Model file for the job. Use its own axes, mm. Face numbers are marked on the shaded views. A direction names the side the tool comes from. Round coordinates to 2 decimals unless told otherwise and drop trailing zeros. Order: outer loops, then holes, each group sorted by start corner. A loop starts at its lowest first (then second) coordinate and runs counter-clockwise, first axis right, second up. Notation, with made-up numbers: (-10.75, 65.25) -> (28.25, 65.25) arc R21 cw to (28.25, 102.25) -> close; hole circle Ø3 at (3, 5). An arc over 180 degrees is marked (long way). Put each result on its own line as item: value. Start each with the question number.
Q1. Cut at C-C, the plane y = -6.25. List the corners of the cut face in (x, z).
Q2. Pull direction Y, two halves, no side cores. Call the marked faces 4, 5 and 6: released by +Y, released by -Y, zero draft, split by the parting line, or undercut.
Q3. Cut at A-A, the plane z = 2.6. State how many separate pieces and enclosed holes the cut face has, and give its area (3 significant figures).
Q4. Flat gauge pins, fed straight in: P1, Ø3.5, axis at x = 4.5, y = 0, coming from the -Z side; P2, Ø3, axis at x = 30.75, y = 0, coming from the +Z side; P3, Ø2, axis at x = 18.5, z = 2, coming from the -Y side; P4, Ø2, axis at y = -10, z = 2.5, coming from the +X side. Where does each tip first touch, or does it go through?
Q5. 3-axis set-ups, long thin cutter, end or side, ignore diameter. For the marked faces 1, 2 and 3: which of +Z, -Z, +X, -X, +Y, -Y reach the whole face in a straight line?
Q6. Cut at B-B, the plane x = 18.5. List the corners of the cut face in (y, z).
Q7. Probe L1, parallel to Y at x = 0, z = 1.85; L2, parallel to X at y = -13, z = 2.95; L3, parallel to Y at x = -11.5, z = 0.6. List the from-to ranges inside material, lowest first.
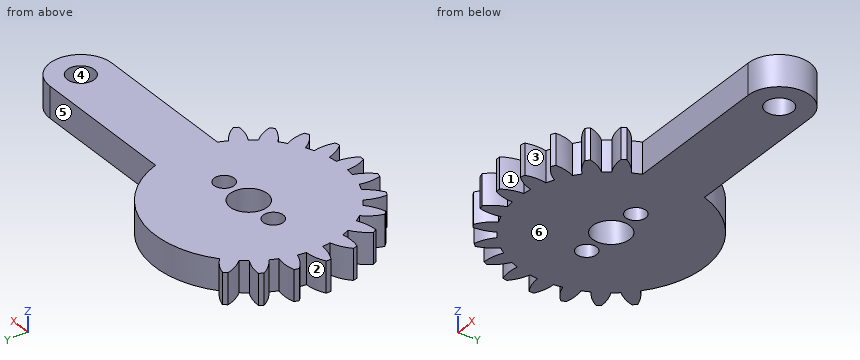
from build123d import *

# Parameters (mm, degrees)
SKETCH1_R           = 1.75
BOSS_EXTRUDE3_DEPTH = 4
SKETCH3_R           = 1.3
SKETCH3_R_2         = 2.4
CUT_EXTRUDE1_DEPTH  = 38.915688046


with BuildPart() as part:
    # Sketch1 → Boss-Extrude3 (new body)
    with BuildSketch(Plane.XY):
        with BuildLine():
            ThreePointArc((11.398526221, 4), (3.187763399, 11.651805204), (-7.774744082, 9.245526186))
            ThreePointArc((-7.774744082, 9.245526186), (-8.865739978, 10.052419077), (-10.123446462, 10.561852666))
            ThreePointArc((-10.123446462, 10.561852666), (-10.344972209, 10.344972209), (-10.561852666, 10.123446462))
            ThreePointArc((-10.561852666, 10.123446462), (-10.052419077, 8.865739978), (-9.245526186, 7.774744082))
            ThreePointArc((-9.245526186, 7.774744082), (-9.583708351, 7.353838062), (-9.90274436, 6.918240682))
            ThreePointArc((-9.90274436, 6.918240682), (-11.16540472, 7.415268848), (-12.51210701, 7.581825517))
            ThreePointArc((-12.51210701, 7.581825517), (-12.669951657, 7.315), (-12.82210701, 7.044889767))
            ThreePointArc((-12.82210701, 7.044889767), (-12.004513558, 5.961889707), (-10.94274436, 5.116907842))
            ThreePointArc((-10.94274436, 5.116907842), (-11.160464753, 4.622815863), (-11.355888976, 4.119488508))
            ThreePointArc((-11.355888976, 4.119488508), (-12.704165582, 4.272780301), (-14.048088143, 4.085109489))
            ThreePointArc((-14.048088143, 4.085109489), (-14.131494839, 3.78652263), (-14.208555951, 3.486235477))
            ThreePointArc((-14.208555951, 3.486235477), (-13.138520279, 2.651746506), (-11.89423259, 2.110362789))
            ThreePointArc((-11.89423259, 2.110362789), (-11.976653925, 1.576756402), (-12.035148524, 1.04))
            ThreePointArc((-12.035148524, 1.04), (-13.377158555, 0.839108838), (-14.626715284, 0.31))
            ThreePointArc((-14.626715284, 0.31), (-14.63, 0), (-14.626715284, -0.31))
            ThreePointArc((-14.626715284, -0.31), (-13.377158555, -0.839108838), (-12.035148524, -1.04))
            ThreePointArc((-12.035148524, -1.04), (-11.976653925, -1.576756402), (-11.89423259, -2.110362789))
            ThreePointArc((-11.89423259, -2.110362789), (-13.138520279, -2.651746506), (-14.208555951, -3.486235477))
            ThreePointArc((-14.208555951, -3.486235477), (-14.131494839, -3.78652263), (-14.048088143, -4.085109489))
            ThreePointArc((-14.048088143, -4.085109489), (-12.704165582, -4.272780301), (-11.355888976, -4.119488508))
            ThreePointArc((-11.355888976, -4.119488508), (-11.160464753, -4.622815863), (-10.94274436, -5.116907842))
            ThreePointArc((-10.94274436, -5.116907842), (-12.004513558, -5.961889707), (-12.82210701, -7.044889767))
            ThreePointArc((-12.82210701, -7.044889767), (-12.669951657, -7.315), (-12.51210701, -7.581825517))
            ThreePointArc((-12.51210701, -7.581825517), (-11.16540472, -7.415268848), (-9.90274436, -6.918240682))
            ThreePointArc((-9.90274436, -6.918240682), (-9.583708351, -7.353838062), (-9.245526186, -7.774744082))
            ThreePointArc((-9.245526186, -7.774744082), (-10.052419077, -8.865739978), (-10.561852666, -10.123446462))
            ThreePointArc((-10.561852666, -10.123446462), (-10.344972209, -10.344972209), (-10.123446462, -10.561852666))
            ThreePointArc((-10.123446462, -10.561852666), (-8.865739978, -10.052419077), (-7.774744082, -9.245526186))
            ThreePointArc((-7.774744082, -9.245526186), (-7.353838062, -9.583708351), (-6.918240682, -9.90274436))
            ThreePointArc((-6.918240682, -9.90274436), (-7.415268848, -11.16540472), (-7.581825517, -12.51210701))
            ThreePointArc((-7.581825517, -12.51210701), (-7.315, -12.669951657), (-7.044889767, -12.82210701))
            ThreePointArc((-7.044889767, -12.82210701), (-5.961889707, -12.004513558), (-5.116907842, -10.94274436))
            ThreePointArc((-5.116907842, -10.94274436), (-4.622815863, -11.160464753), (-4.119488508, -11.355888976))
            ThreePointArc((-4.119488508, -11.355888976), (-4.272780301, -12.704165582), (-4.085109489, -14.048088143))
            ThreePointArc((-4.085109489, -14.048088143), (-3.78652263, -14.131494839), (-3.486235477, -14.208555951))
            ThreePointArc((-3.486235477, -14.208555951), (-2.651746506, -13.138520279), (-2.110362789, -11.89423259))
            ThreePointArc((-2.110362789, -11.89423259), (-1.576756402, -11.976653925), (-1.04, -12.035148524))
            ThreePointArc((-1.04, -12.035148524), (-0.839108838, -13.377158555), (-0.31, -14.626715284))
            ThreePointArc((-0.31, -14.626715284), (0, -14.63), (0.31, -14.626715284))
            ThreePointArc((0.31, -14.626715284), (0.839108838, -13.377158555), (1.04, -12.035148524))
            ThreePointArc((1.04, -12.035148524), (1.576756402, -11.976653925), (2.110362789, -11.89423259))
            ThreePointArc((2.110362789, -11.89423259), (2.651746506, -13.138520279), (3.486235477, -14.208555951))
            ThreePointArc((3.486235477, -14.208555951), (3.78652263, -14.131494839), (4.085109489, -14.048088143))
            ThreePointArc((4.085109489, -14.048088143), (4.272780301, -12.704165582), (4.119488508, -11.355888976))
            ThreePointArc((4.119488508, -11.355888976), (4.622815863, -11.160464753), (5.116907842, -10.94274436))
            ThreePointArc((5.116907842, -10.94274436), (5.961889707, -12.004513558), (7.044889767, -12.82210701))
            ThreePointArc((7.044889767, -12.82210701), (7.315, -12.669951657), (7.581825517, -12.51210701))
            ThreePointArc((7.581825517, -12.51210701), (7.415268848, -11.16540472), (6.918240682, -9.90274436))
            ThreePointArc((6.918240682, -9.90274436), (7.353838062, -9.583708351), (7.774744082, -9.245526186))
            ThreePointArc((7.774744082, -9.245526186), (8.865739978, -10.052419077), (10.123446462, -10.561852666))
            ThreePointArc((10.123446462, -10.561852666), (10.344972209, -10.344972209), (10.561852666, -10.123446462))
            ThreePointArc((10.561852666, -10.123446462), (10.052419077, -8.865739978), (9.245526186, -7.774744082))
            ThreePointArc((9.245526186, -7.774744082), (9.583708351, -7.353838062), (9.90274436, -6.918240682))
            ThreePointArc((9.90274436, -6.918240682), (11.16540472, -7.415268848), (12.51210701, -7.581825517))
            ThreePointArc((12.51210701, -7.581825517), (12.669951657, -7.315), (12.82210701, -7.044889767))
            ThreePointArc((12.82210701, -7.044889767), (12.004513558, -5.961889707), (10.94274436, -5.116907842))
            ThreePointArc((10.94274436, -5.116907842), (11.184585981, -4.564146845), (11.398526221, -4))
            Line((11.398526221, -4), (30.75, -4))
            ThreePointArc((30.75, -4), (34.75, 0), (30.75, 4))
            Line((30.75, 4), (11.398526221, 4))
        make_face()
        Circle(SKETCH1_R, mode=Mode.SUBTRACT)
        with Locations((30.75, 0)):
            Circle(SKETCH1_R, mode=Mode.SUBTRACT)
    extrude(amount=BOSS_EXTRUDE3_DEPTH)

    # Sketch3 → Cut-Extrude1 (cut, through all)
    with BuildSketch(Plane.XY.offset(4)):
        with Locations((4.5, 0)):
            Circle(SKETCH3_R)
        with Locations((-4.5, 0)):
            Circle(SKETCH3_R)
        Circle(SKETCH3_R_2)
    extrude(amount=-CUT_EXTRUDE1_DEPTH, mode=Mode.SUBTRACT)


solid = part.part
Ans:
1. outline: (-12.27, 0) -> (12.27, 0) -> (12.27, 4) -> (-12.27, 4) -> close
2. face 4: undercut
2. face 5: released by +Y
2. face 6: zero draft
3. separate pieces: 1
3. enclosed holes: 4
3. area: 653 mm^2
4. P1: stops at z = 0
4. P2: passes through
4. P3: stops at y = -4
4. P4: stops at x = 10.56
5. face 1: +Z, -Z, -Y
5. face 2: +Z, -Z, -X
5. face 3: +Z, -Z
6. outline: (-4, 0) -> (4, 0) -> (4, 4) -> (-4, 4) -> close
7. L1: y = -14.63 to -2.4, 2.4 to 12.08
7. L2: x = -4.26 to -2.57, -0.93 to 0.93, 2.57 to 4.26
7. L3: y = -7.49 to -5.51, -4.15 to 4.15, 5.51 to 7.49
